Here's how the part is built. I have some questions about the finished solid (model axes, mm). Face numbers are marked on the shaded views. Coordinates: 2 decimals unless noted, no trailing zeros. Order: outer loops, then holes, each group sorted by start corner. A loop starts at its lowest first (then second) coordinate and runs counter-clockwise, first axis right, second up. Notation, with made-up numbers: (64.25, 86.25) - (80.25, 86.25) arc R12 cw to (80.25, 104.25) - close; hole circle Ø8 at (43, 61). An arc over 180 degrees is marked (long way). Use CSV: the item, a comma, the result in double quotes. Start each with the question number.
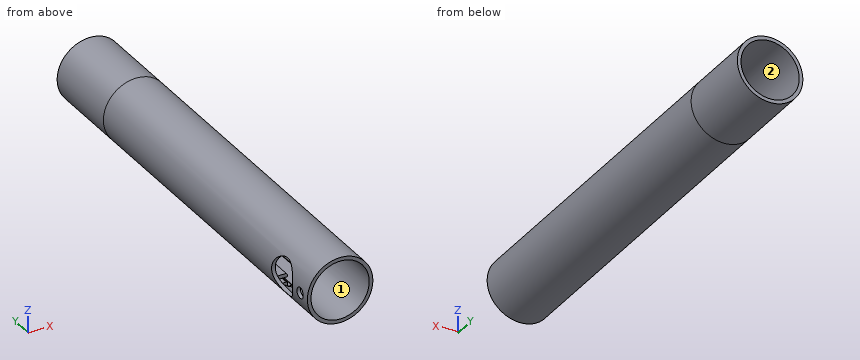
from build123d import *

# Parameters (mm, degrees)
F3_R      = 4.5
F4_DEPTH  = 39.5
F8_DEPTH  = 39.5
F6_R      = 4.5
F6_R_2    = 4
F9_DEPTH  = 9
F7_R      = 4.5
F7_R_2    = 4
F10_DEPTH = 11
F11_R     = 2.5
F11_R_2   = 0.75
F12_DEPTH = 4.501


# Not quite as in the source:
# - ends of sketch curves that miss each other by under 0.0002 mm in the source are joined


with BuildPart() as f4:
    # F3 (on Front) → F4 (new body)
    with BuildSketch(Plane.XZ):
        Circle(F3_R)
    extrude(amount=F4_DEPTH)

    # F5 (on face) → F8 (cut, through all)
    with BuildSketch(Plane.XZ.offset(39.5)):
        with BuildLine():
            Line((-1.25, -3.8), (0, -3.8))
            Line((0, -3.8), (1.25, -3.8))
            Line((1.25, -3.8), (1.25, -3.7))
            ThreePointArc((1.25, -3.7), (1.3085786438, -3.5585786438), (1.45, -3.5))
            Line((1.45, -3.5), (2, -3.5))
            Line((2, -3.5), (2, -3.05))
            ThreePointArc((2, -3.05), (2.0585786438, -2.9085786438), (2.2, -2.85))
            Line((2.2, -2.85), (3.15, -2.85))
            Line((3.15, -2.85), (3.15, -2.15))
            Line((3.15, -2.15), (2.2, -2.15))
            ThreePointArc((2.2, -2.15), (2.0585786438, -2.0914213562), (2, -1.95))
            Line((2, -1.95), (2, -1.887459))
            ThreePointArc((2, -1.887459), (2.1033535752, -1.771554046), (2.2, -1.65))
            Line((2.2, -1.65), (3.75, -1.65))
            Line((3.75, -1.65), (3.75, 0))
            Line((3.75, 0), (3.75, 1.65))
            Line((3.75, 1.65), (2.2, 1.65))
            ThreePointArc((2.2, 1.65), (2.1033535752, 1.771554046), (1.9999998047, 1.8874588157))
            Line((1.9999998047, 1.8874588157), (2, 1.95))
            ThreePointArc((2, 1.95), (2.0585786438, 2.0914213562), (2.2, 2.15))
            Line((2.2, 2.15), (3.15, 2.15))
            Line((3.15, 2.15), (3.15, 2.85))
            Line((3.15, 2.85), (2.2, 2.85))
            ThreePointArc((2.2, 2.85), (2.0585786438, 2.9085786438), (2, 3.05))
            Line((2, 3.05), (2, 3.5))
            Line((2, 3.5), (1.45, 3.5))
            ThreePointArc((1.45, 3.5), (1.3085786438, 3.5585786438), (1.25, 3.7))
            Line((1.25, 3.7), (1.25, 3.8))
            Line((1.25, 3.8), (0, 3.8))
            Line((0, 3.8), (-1.25, 3.8))
            Line((-1.25, 3.8), (-1.25, 3.7))
            ThreePointArc((-1.25, 3.7), (-1.3085786438, 3.5585786438), (-1.45, 3.5))
            Line((-1.45, 3.5), (-2, 3.5))
            Line((-2, 3.5), (-2, 3.05))
            ThreePointArc((-2, 3.05), (-2.0585786438, 2.9085786438), (-2.2, 2.85))
            Line((-2.2, 2.85), (-3.15, 2.85))
            Line((-3.15, 2.85), (-3.15, 2.15))
            Line((-3.15, 2.15), (-2.2, 2.15))
            ThreePointArc((-2.2, 2.15), (-2.0585786438, 2.0914213562), (-2, 1.95))
            Line((-2, 1.95), (-2, 1.887459))
            ThreePointArc((-2, 1.887459), (-2.1033535752, 1.771554046), (-2.2, 1.65))
            Line((-2.2, 1.65), (-3.75, 1.65))
            Line((-3.75, 1.65), (-3.75, 0))
            Line((-3.75, 0), (-3.75, -1.65))
            Line((-3.75, -1.65), (-2.2, -1.65))
            ThreePointArc((-2.2, -1.65), (-2.1033535752, -1.771554046), (-1.9999998047, -1.8874588157))
            Line((-1.9999998047, -1.8874588157), (-2, -1.95))
            ThreePointArc((-2, -1.95), (-2.0585786438, -2.0914213562), (-2.2, -2.15))
            Line((-2.2, -2.15), (-3.15, -2.15))
            Line((-3.15, -2.15), (-3.15, -2.85))
            Line((-3.15, -2.85), (-2.2, -2.85))
            ThreePointArc((-2.2, -2.85), (-2.0585786438, -2.9085786438), (-2, -3.05))
            Line((-2, -3.05), (-2, -3.5))
            Line((-2, -3.5), (-1.45, -3.5))
            ThreePointArc((-1.45, -3.5), (-1.3085786438, -3.5585786438), (-1.25, -3.7))
            Line((-1.25, -3.7), (-1.25, -3.8))
        make_face()
    extrude(amount=-F8_DEPTH, mode=Mode.SUBTRACT)

    # F6 (on face) → F9 (join)
    with BuildSketch(Plane.XZ.offset(39.5)):
        Circle(F6_R)
        Circle(F6_R_2, mode=Mode.SUBTRACT)
    extrude(amount=F9_DEPTH)

    # F7 (on face) → F10 (join)
    with BuildSketch(Plane(origin=(0, 0, 0), x_dir=(-1, 0, 0), z_dir=(0, 1, 0))):
        Circle(F7_R)
        Circle(F7_R_2, mode=Mode.SUBTRACT)
    extrude(amount=F10_DEPTH)

    # F11 (on Right) → F12 (cut, through all)
    with BuildSketch(Plane.YZ):
        with Locations((-42.5, 0)):
            Circle(F11_R)
        with Locations((-46.75, 0)):
            Circle(F11_R_2)
    extrude(amount=-F12_DEPTH, mode=Mode.SUBTRACT)


solid = f4.part
Item 1: Please list where these lines run through material, in increasing order: line 1 along Z through (x, y) = (-2.5, -11); line 2 along X through (y, z) = (-18, 0.25); line 3 along Z through (x, y) = (2.75, -34.5). Write a range as from..to.
Item 2: Suppose I cut it at D-D on y = -42.5. Write out the boundary of the cut face in (x, z).
Item 3: Suppose I cut it at B-B on z = 0. Write out the boundary of the cut face in (x, y), then the cut area to 3 significant figures.
Item 4: For pin 1 Ø1.5 at (x, y) = (-3, 2) entering from +Z; pin 2 Ø0.8 at (y, z) = (-12.5, 2.5) entering from +X; pin 3 Ø2 at (x, y) = (2.5, -15.5) entering from -Z, each with a flat end and sliding along its axis, tell me the tip position at first contact or that it passes through.
Item 5: Suppose I cut it at A-A on x = 0. Write out the boundary of the cut face in (y, z), then the cut area to 3 significant figures.
Item 6: We'd pull the mould along Z, two halves only. Please class the marked faces 1 and 2: released by +Z, released by -Z, zero draft, split by the parting line, or undercut.
Item 7: Suppose I cut it at C-C on y = 5. Write out the boundary of the cut face in (x, z).
Here are the results:
1,line 1,"-3.74..-2.85, -2.15..-1.65, 1.65..2.15, 2.85..3.74"
1,line 2,"-4.49..-3.75, 3.75..4.49"
1,line 3,"-3.56..-2.85, -2.15..-1.65, 1.65..2.15, 2.85..3.56"
2,outline,"(-3.74, -2.5) arc R4.5 ccw (long way) to (-3.74, 2.5) - (-3.12, 2.5) arc R4 cw (long way) to (-3.12, -2.5) - close"
3,outline,"(-4.5, -48.5) - (-4, -48.5) - (-4, -47.5) - (-4.5, -47.5) - close; (-4.5, -46) - (-4, -46) - (-4, -45) - (-4.5, -45) - close; (-4.5, -40) - (-4, -40) - (-4, -39.5) - (-3.75, -39.5) - (-3.75, 0) - (-4, 0) - (-4, 11) - (-4.5, 11) - close; (3.75, -39.5) - (4, -39.5) - (4, -48.5) - (4.5, -48.5) - (4.5, 11) - (4, 11) - (4, 0) - (3.75, 0) - close"
3,area,"76.0 mm^2"
4,pin 1,"z = 3.9"
4,pin 2,"x = 3.98"
4,pin 3,"z = -4.24"
5,outline,"(-48.5, -4.5) - (11, -4.5) - (11, -4) - (0, -4) - (0, -3.8) - (-39.5, -3.8) - (-39.5, -4) - (-48.5, -4) - close; (-48.5, 4) - (-39.5, 4) - (-39.5, 3.8) - (0, 3.8) - (0, 4) - (11, 4) - (11, 4.5) - (-48.5, 4.5) - close"
5,area,"75.3 mm^2"
6,face 1,"undercut"
6,face 2,"undercut"
7,outline,"circle Ø9 at (0, 0); hole circle Ø8 at (0, 0)"
